The model under review builds one solid part; all positions refer to its coordinate system, in mm. Round coordinates to 2 decimals unless told otherwise and drop trailing zeros. Order: outer loops, then holes, each group sorted by start corner. A loop starts at its lowest first (then second) coordinate and runs counter-clockwise, first axis right, second up. Notation, with made-up numbers: M 49.5,67 L 89.5,67 A16 cw 89.5,95 Z; hole C 60,20.25 d2. An arc over 180 degrees is marked long. Use a Markdown table: item, result. Add a question column.
1. Insertion check: P1, Ø4, axis at x = -1.5, z = 71, coming from the +Y side. The pin has a flat end and moves straight along its axis. Give the tip position at first contact, or say it passes through.
2. To check wall thickness, follow probe 1 along Y at (x, z) = (13.25, 89); probe 2 along X at (y, z) = (1, 93); probe 3 along X at (y, z) = (-5.5, 30.5). State the ranges of each line that lie inside material, in increasing order.
3. Consider section B-B on z = 12.5. Count the separate pieces of the cut face and the enclosed holes in it, then the cut area to 3 significant figures.
4. Consider section A-A on x = -1.5. State the section outline as (y, z) points.
from build123d import *

# Parameters (mm, degrees)
SKETCH_1_R      = 3.4
EXTRUDE_1_DEPTH = 100


with BuildPart() as part:
    # 草图1 → 凸台-拉伸1 (new body)
    with BuildSketch(Plane.XY):
        with BuildLine():
            Line((5.859616846, 16.034137905), (12.959616847, 16.034137905))
            ThreePointArc((12.959616847, 16.034137905), (14.7273838, 15.301904858), (15.459616847, 13.534137905))
            Line((15.459616847, 13.534137905), (15.459616847, 6.434137905))
            ThreePointArc((15.459616847, 6.434137905), (15.371748881, 6.222005871), (15.159616847, 6.134137905))
            Line((15.159616847, 6.134137905), (14.759616847, 6.134137905))
            ThreePointArc((14.759616847, 6.134137905), (14.547484812, 6.046269939), (14.459616847, 5.834137905))
            Line((14.459616847, 5.834137905), (14.459616847, 5.434137905))
            ThreePointArc((14.459616847, 5.434137905), (14.371748881, 5.222005871), (14.159616847, 5.134137905))
            Line((14.159616847, 5.134137905), (13.759616847, 5.134137905))
            ThreePointArc((13.759616847, 5.134137905), (13.547484812, 5.222005871), (13.459616847, 5.434137905))
            Line((13.459616847, 5.434137905), (13.459616847, 8.984137905))
            ThreePointArc((13.459616847, 8.984137905), (13.371748881, 9.196269939), (13.159616847, 9.284137905))
            Line((13.159616847, 9.284137905), (10.248094478, 9.284137905))
            ThreePointArc((10.248094478, 9.284137905), (10.133289448, 9.261301765), (10.035962443, 9.196269939))
            Line((10.035962443, 9.196269939), (6.347484812, 5.507792308))
            ThreePointArc((6.347484812, 5.507792308), (6.282452987, 5.410465304), (6.259616847, 5.295660274))
            Line((6.259616847, 5.295660274), (6.259616847, 1.784137905))
            Line((6.259616847, 1.784137905), (5.826604145, 1.034137905))
            Line((5.826604145, 1.034137905), (6.259616847, 0.284137905))
            Line((6.259616847, 0.284137905), (6.259616847, -3.227384464))
            ThreePointArc((6.259616847, -3.227384464), (6.282452987, -3.342189494), (6.347484812, -3.439516498))
            Line((6.347484812, -3.439516498), (10.035962443, -7.127994129))
            ThreePointArc((10.035962443, -7.127994129), (10.133289448, -7.193025955), (10.248094478, -7.215862095))
            Line((10.248094478, -7.215862095), (13.159616847, -7.215862095))
            ThreePointArc((13.159616847, -7.215862095), (13.371748881, -7.127994129), (13.459616847, -6.915862095))
            Line((13.459616847, -6.915862095), (13.459616847, -3.365862095))
            ThreePointArc((13.459616847, -3.365862095), (13.547484812, -3.153730061), (13.759616847, -3.065862095))
            Line((13.759616847, -3.065862095), (14.159616847, -3.065862095))
            ThreePointArc((14.159616847, -3.065862095), (14.371748881, -3.153730061), (14.459616847, -3.365862095))
            Line((14.459616847, -3.365862095), (14.459616847, -3.765862095))
            ThreePointArc((14.459616847, -3.765862095), (14.547484812, -3.977994129), (14.759616847, -4.065862095))
            Line((14.759616847, -4.065862095), (15.159616847, -4.065862095))
            ThreePointArc((15.159616847, -4.065862095), (15.371748881, -4.153730061), (15.459616847, -4.365862095))
            Line((15.459616847, -4.365862095), (15.459616847, -11.465862095))
            ThreePointArc((15.459616847, -11.465862095), (14.7273838, -13.233629048), (12.959616847, -13.965862095))
            Line((12.959616847, -13.965862095), (-12.040383153, -13.965862095))
            ThreePointArc((-12.040383153, -13.965862095), (-13.808150106, -13.233629048), (-14.540383153, -11.465862095))
            Line((-14.540383153, -11.465862095), (-14.540383153, 13.534137905))
            ThreePointArc((-14.540383153, 13.534137905), (-13.808150106, 15.301904858), (-12.040383153, 16.034137905))
            Line((-12.040383153, 16.034137905), (-4.940383153, 16.034137905))
            ThreePointArc((-4.940383153, 16.034137905), (-4.728251119, 15.94626994), (-4.640383153, 15.734137905))
            Line((-4.640383153, 15.734137905), (-4.640383153, 15.334137905))
            ThreePointArc((-4.640383153, 15.334137905), (-4.552515188, 15.122005871), (-4.340383153, 15.034137905))
            Line((-4.340383153, 15.034137905), (-3.940383153, 15.034137905))
            ThreePointArc((-3.940383153, 15.034137905), (-3.728251119, 14.946269939), (-3.640383153, 14.734137905))
            Line((-3.640383153, 14.734137905), (-3.640383153, 14.334137905))
            ThreePointArc((-3.640383153, 14.334137905), (-3.728251119, 14.122005871), (-3.940383153, 14.034137905))
            Line((-3.940383153, 14.034137905), (-7.490383153, 14.034137905))
            ThreePointArc((-7.490383153, 14.034137905), (-7.702515188, 13.946269939), (-7.790383153, 13.734137905))
            Line((-7.790383153, 13.734137905), (-7.790383153, 10.822615536))
            ThreePointArc((-7.790383153, 10.822615536), (-7.767547013, 10.707810506), (-7.702515188, 10.610483502))
            Line((-7.702515188, 10.610483502), (-4.014037557, 6.922005871))
            ThreePointArc((-4.014037557, 6.922005871), (-3.916710552, 6.856974045), (-3.801905522, 6.834137905))
            Line((-3.801905522, 6.834137905), (-0.290383153, 6.834137905))
            Line((-0.290383153, 6.834137905), (0.459616847, 6.401125203))
            Line((0.459616847, 6.401125203), (1.209616847, 6.834137905))
            Line((1.209616847, 6.834137905), (4.721139216, 6.834137905))
            ThreePointArc((4.721139216, 6.834137905), (4.835944245, 6.856974045), (4.93327125, 6.922005871))
            Line((4.93327125, 6.922005871), (8.621748881, 10.610483502))
            ThreePointArc((8.621748881, 10.610483502), (8.686780706, 10.707810507), (8.709616847, 10.822615536))
            Line((8.709616847, 10.822615536), (8.709616847, 13.734137905))
            ThreePointArc((8.709616847, 13.734137905), (8.621748881, 13.946269939), (8.409616847, 14.034137905))
            Line((8.409616847, 14.034137905), (4.859616847, 14.034137905))
            ThreePointArc((4.859616847, 14.034137905), (4.647484812, 14.122005871), (4.559616847, 14.334137905))
            Line((4.559616847, 14.334137905), (4.559616847, 14.734137905))
            ThreePointArc((4.559616847, 14.734137905), (4.647484812, 14.946269939), (4.859616847, 15.034137905))
            Line((4.859616847, 15.034137905), (5.259616847, 15.034137905))
            ThreePointArc((5.259616847, 15.034137905), (5.471748881, 15.122005871), (5.559616847, 15.334137905))
            Line((5.559616847, 15.334137905), (5.559616847, 15.734137905))
            ThreePointArc((5.559616847, 15.734137905), (5.647484812, 15.94626994), (5.859616846, 16.034137905))
        make_face()
        with Locations((0.459616847, 1.034137905)):
            Circle(SKETCH_1_R, mode=Mode.SUBTRACT)
        with BuildLine():
            Line((8.409616847, -11.965862095), (-7.490383153, -11.965862095))
            ThreePointArc((-7.490383153, -11.965862095), (-7.702515188, -11.877994129), (-7.790383153, -11.665862095))
            Line((-7.790383153, -11.665862095), (-7.790383153, -8.754339726))
            ThreePointArc((-7.790383153, -8.754339726), (-7.767547013, -8.639534696), (-7.702515188, -8.542207692))
            Line((-7.702515188, -8.542207692), (-4.014037557, -4.853730061))
            ThreePointArc((-4.014037557, -4.853730061), (-3.916710552, -4.788698235), (-3.801905522, -4.765862095))
            Line((-3.801905522, -4.765862095), (-0.290383153, -4.765862095))
            Line((-0.290383153, -4.765862095), (0.459616847, -4.332849393))
            Line((0.459616847, -4.332849393), (1.209616847, -4.765862095))
            Line((1.209616847, -4.765862095), (4.721139216, -4.765862095))
            ThreePointArc((4.721139216, -4.765862095), (4.835944245, -4.788698235), (4.93327125, -4.853730061))
            Line((4.93327125, -4.853730061), (8.621748881, -8.542207692))
            ThreePointArc((8.621748881, -8.542207692), (8.686780706, -8.639534696), (8.709616847, -8.754339726))
            Line((8.709616847, -8.754339726), (8.709616847, -11.665862095))
            ThreePointArc((8.709616847, -11.665862095), (8.621748881, -11.877994129), (8.409616847, -11.965862095))
        make_face(mode=Mode.SUBTRACT)
        with BuildLine():
            Line((-10.290383153, -8.715862095), (-12.190383153, -8.715862095))
            ThreePointArc((-12.190383153, -8.715862095), (-12.897489934, -9.008755314), (-13.190383153, -9.715862095))
            Line((-13.190383153, -9.715862095), (-13.190383153, -11.615862095))
            ThreePointArc((-13.190383153, -11.615862095), (-12.897489934, -12.322968876), (-12.190383153, -12.615862095))
            Line((-12.190383153, -12.615862095), (-10.290383153, -12.615862095))
            ThreePointArc((-10.290383153, -12.615862095), (-9.583276372, -12.322968876), (-9.290383153, -11.615862095))
            Line((-9.290383153, -11.615862095), (-9.290383153, -9.715862095))
            ThreePointArc((-9.290383153, -9.715862095), (-9.583276372, -9.008755314), (-10.290383153, -8.715862095))
        make_face(mode=Mode.SUBTRACT)
        with BuildLine():
            Line((-9.290383153, 13.684137905), (-9.290383153, 11.784137905))
            ThreePointArc((-9.290383153, 11.784137905), (-9.583276372, 11.077031124), (-10.290383153, 10.784137905))
            Line((-10.290383153, 10.784137905), (-12.190383153, 10.784137905))
            ThreePointArc((-12.190383153, 10.784137905), (-12.897489934, 11.077031124), (-13.190383153, 11.784137905))
            Line((-13.190383153, 11.784137905), (-13.190383153, 13.684137905))
            ThreePointArc((-13.190383153, 13.684137905), (-12.897489934, 14.391244686), (-12.190383153, 14.684137905))
            Line((-12.190383153, 14.684137905), (-10.290383153, 14.684137905))
            ThreePointArc((-10.290383153, 14.684137905), (-9.583276372, 14.391244686), (-9.290383153, 13.684137905))
        make_face(mode=Mode.SUBTRACT)
        with BuildLine():
            Line((13.109616847, 10.784137905), (11.209616847, 10.784137905))
            ThreePointArc((11.209616847, 10.784137905), (10.502510066, 11.077031124), (10.209616847, 11.784137905))
            Line((10.209616847, 11.784137905), (10.209616847, 13.684137905))
            ThreePointArc((10.209616847, 13.684137905), (10.502510066, 14.391244686), (11.209616847, 14.684137905))
            Line((11.209616847, 14.684137905), (13.109616847, 14.684137905))
            ThreePointArc((13.109616847, 14.684137905), (13.816723628, 14.391244686), (14.109616847, 13.684137905))
            Line((14.109616847, 13.684137905), (14.109616847, 11.784137905))
            ThreePointArc((14.109616847, 11.784137905), (13.816723628, 11.077031124), (13.109616847, 10.784137905))
        make_face(mode=Mode.SUBTRACT)
        with BuildLine():
            Line((-5.340383153, 5.295660274), (-5.340383153, 1.784137905))
            Line((-5.340383153, 1.784137905), (-4.907370451, 1.034137905))
            Line((-4.907370451, 1.034137905), (-5.340383153, 0.284137905))
            Line((-5.340383153, 0.284137905), (-5.340383153, -3.227384464))
            ThreePointArc((-5.340383153, -3.227384464), (-5.363219294, -3.342189494), (-5.428251119, -3.439516498))
            Line((-5.428251119, -3.439516498), (-9.11672875, -7.127994129))
            ThreePointArc((-9.11672875, -7.127994129), (-9.214055755, -7.193025955), (-9.328860784, -7.215862095))
            Line((-9.328860784, -7.215862095), (-12.240383153, -7.215862095))
            ThreePointArc((-12.240383153, -7.215862095), (-12.452515188, -7.127994129), (-12.540383153, -6.915862095))
            Line((-12.540383153, -6.915862095), (-12.540383153, 8.984137905))
            ThreePointArc((-12.540383153, 8.984137905), (-12.452515188, 9.196269939), (-12.240383153, 9.284137905))
            Line((-12.240383153, 9.284137905), (-9.328860784, 9.284137905))
            ThreePointArc((-9.328860784, 9.284137905), (-9.214055755, 9.261301765), (-9.11672875, 9.196269939))
            Line((-9.11672875, 9.196269939), (-5.428251119, 5.507792308))
            ThreePointArc((-5.428251119, 5.507792308), (-5.363219294, 5.410465304), (-5.340383153, 5.295660274))
        make_face(mode=Mode.SUBTRACT)
        with BuildLine():
            Line((14.109616847, -11.615862095), (14.109616847, -9.715862095))
            ThreePointArc((14.109616847, -9.715862095), (13.816723628, -9.008755314), (13.109616847, -8.715862095))
            Line((13.109616847, -8.715862095), (11.209616847, -8.715862095))
            ThreePointArc((11.209616847, -8.715862095), (10.502510066, -9.008755314), (10.209616847, -9.715862095))
            Line((10.209616847, -9.715862095), (10.209616847, -11.615862095))
            ThreePointArc((10.209616847, -11.615862095), (10.502510066, -12.322968876), (11.209616847, -12.615862095))
            Line((11.209616847, -12.615862095), (13.109616847, -12.615862095))
            ThreePointArc((13.109616847, -12.615862095), (13.816723628, -12.322968876), (14.109616847, -11.615862095))
        make_face(mode=Mode.SUBTRACT)
    extrude(amount=EXTRUDE_1_DEPTH)


solid = part.part
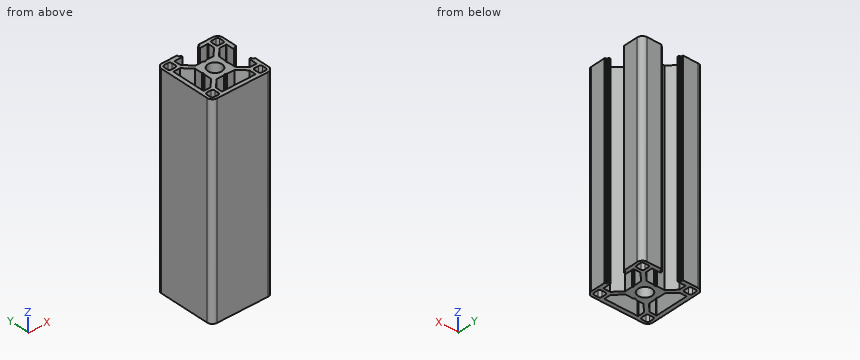
Answer block:
| question | item | result |
|---|---|---|
| 1 | P1 | y = 6.83 |
| 2 | probe 1 | -13.95 to -12.61, -8.73 to -7.2, 9.27 to 10.79, 14.67 to 16.02 |
| 2 | probe 2 | -14.54 to -12.54, -4.93 to -2.94, 3.86 to 5.85 |
| 2 | probe 3 | -14.54 to -12.54, -7.49 to -4.66, 5.58 to 8.41, 13.46 to 15.46 |
| 3 | separate pieces | 1 |
| 3 | enclosed holes | 7 |
| 3 | area | 347 mm^2 |
| 4 | outline | M -13.97,0 L -11.97,0 L -11.97,100 L -13.97,100 Z; M -4.77,0 L -1.74,0 L -1.74,100 L -4.77,100 Z; M 3.81,0 L 6.83,0 L 6.83,100 L 3.81,100 Z |
